from build123d import *

# Parameters (mm, degrees)
F5_R     = 30.5
F5_W     = 20
F5_H     = 15
F0_DEPTH = 80
F2_DEPTH = 1
F4_DEPTH = 1


with BuildPart() as f0:
    # F5 (on Top) → F0 (new body)
    with BuildSketch(Plane.XY):
        with BuildLine():
            ThreePointArc((-99, 0), (-66, 33), (-33, 0))
            Line((-33, 0), (-33, 50))
            Line((-33, 50), (-79, 50))
            Line((-79, 50), (-79, 35))
            Line((-79, 35), (-99, 35))
            Line((-99, 35), (-99, 0))
        make_face()
        with BuildLine():
            ThreePointArc((-99, 0), (-66, -33), (-33, 0))
            ThreePointArc((-33, 0), (-66, 33), (-99, 0))
        make_face()
        with Locations((-66, 0)):
            Circle(F5_R, mode=Mode.SUBTRACT)
        with Locations((-89, 42.5)):
            Rectangle(F5_W, F5_H)
    extrude(amount=F0_DEPTH)

    # F1 (on face) → F2 (join)
    with BuildSketch(Plane.YZ.offset(-33)):
        Polygon((33.663927, 32.829516), (33.663927, 57.098736), (2.563593, 75.054523), (2.563593, 51.653499), (2.563593, 14.865377), (18.11376, 5.887484), (19.11376, 6.464834), (33.663927, 14.865377), (33.663927, 15.595676), align=None)
        Polygon((4.563593, 51.165515), (4.563593, 71.590421), (31.663927, 55.944036), (31.663927, 53.944036), (31.663927, 46.022312), (31.663927, 43.27108), (31.663927, 32.829516), (31.663927, 16.020077), (18.11376, 8.196885), (4.563593, 16.020077), (4.563593, 32.829516), (4.563593, 35.912469), (4.563593, 36.259414), (4.563593, 38.259414), (4.563593, 49.165515), align=None, mode=Mode.SUBTRACT)
        Polygon((14.651485, 52.944283), (4.563593, 51.165515), (4.563593, 49.165515), (31.663927, 53.944036), (31.663927, 55.944036), (16.651485, 53.296937), align=None)
        Polygon((14.651485, 60.74453), (14.651485, 52.944283), (16.651485, 53.296937), (16.651485, 60.74453), (15.651485, 61.32188), align=None)
        Polygon((17.873782, 38.259414), (4.563593, 35.912469), (4.563593, 32.829516), (19.873782, 35.529115), (19.873782, 46.225284), (18.873782, 46.802635), (17.873782, 46.225284), align=None)
        Polygon((31.663927, 43.27108), (31.663927, 46.022312), (23.782982, 38.337872), (24.068827, 37.214549), (25.17923, 36.905919), align=None)
        Polygon((31.663927, 32.829516), (31.663927, 43.27108), (25.17923, 36.905919), (24.068827, 37.214549), align=None)
        Polygon((21.413582, 22.519643), (21.413582, 26.32995), (18.11376, 28.235103), (14.813938, 26.32995), (14.813938, 22.519643), (18.11376, 20.61449), align=None)
    extrude(amount=F2_DEPTH)

    # F3 (on face) → F4 (join)
    with BuildSketch(Plane(origin=(-99, 0, 0), x_dir=(0, -1, 0), z_dir=(-1, 0, 0))):
        Polygon((-33.316614, 46.639109), (-33.316614, 22.369889), (-2.216279, 4.414102), (-2.216279, 27.815126), (-2.216279, 64.603248), (-17.766446, 73.581141), (-18.766446, 73.003791), (-33.316614, 64.603248), (-33.316614, 63.872949), align=None)
        Polygon((-4.216279, 28.303109), (-4.216279, 7.878204), (-31.316614, 23.524589), (-31.316614, 25.524589), (-31.316614, 33.446313), (-31.316614, 36.197545), (-31.316614, 46.639109), (-31.316614, 63.448548), (-17.766446, 71.27174), (-4.216279, 63.448548), (-4.216279, 46.639109), (-4.216279, 43.556156), (-4.216279, 43.209211), (-4.216279, 41.209211), (-4.216279, 30.303109), align=None, mode=Mode.SUBTRACT)
        Polygon((-17.526468, 41.209211), (-4.216279, 43.556156), (-4.216279, 46.639109), (-19.526468, 43.939509), (-19.526468, 33.243341), (-18.526468, 32.66599), (-17.526468, 33.243341), align=None)
        Polygon((-31.316614, 36.197545), (-31.316614, 33.446313), (-23.435668, 41.130753), (-23.721513, 42.254076), (-24.831917, 42.562706), align=None)
        Polygon((-31.316614, 46.639109), (-31.316614, 36.197545), (-24.831917, 42.562706), (-23.721513, 42.254076), align=None)
        Polygon((-21.066269, 56.948982), (-21.066269, 53.138675), (-17.766446, 51.233521), (-14.466624, 53.138675), (-14.466624, 56.948982), (-17.766446, 58.854135), align=None)
        Polygon((-14.304171, 26.524342), (-4.216279, 28.303109), (-4.216279, 30.303109), (-31.316614, 25.524589), (-31.316614, 23.524589), (-16.304171, 26.171688), align=None)
        Polygon((-14.304171, 18.724095), (-14.304171, 26.524342), (-16.304171, 26.171688), (-16.304171, 18.724095), (-15.304171, 18.146745), align=None)
    extrude(amount=F4_DEPTH)


solid = f0.part
For this review, take the finished solid that the model builds, in its own axes (mm). A direction names the side the tool comes from. Coordinates: 2 decimals unless noted, no trailing zeros. Loops run counter-clockwise (first coordinate to the right, second up) from the corner with the lowest first, then second, coordinate; pieces in that order, holes last. Notation, with made-up numbers: (16.5, -9.5) - (38.5, -9.5) arc R21 ccw to (38.5, -1.5) - close; hole circle Ø2 at (-16.5, -21.5). An arc over 180 degrees is marked (long way). Return JSON: item names as keys, results as strings.
Item 1: For faces 1 (the flat face through (-32.51, 18.33, 65.95)), 2 (the flat face through (-99.49, 23.92, 24.83)), 3 (the flat face through (-32.51, 12.11, 34.16)), list the 3-axis set-ups (+Z, -Z, +X, -X, +Y, -Y) from which the entire face can be reached by the end or side of a thin tool; tool diameter is ignored.
Determined:
{"face 1": "+Z, +X, +Y", "face 2": "-X", "face 3": "+X"}
Item 2: Take a section at B-B (x = -75.5). Give the boundary of the cut face in (y, z).
Determined:
{"outline": "(-31.6, 0) - (-28.98, 0) - (-28.98, 80) - (-31.6, 80) - close; (28.98, 0) - (50, 0) - (50, 80) - (28.98, 80) - close"}
Item 3: Insertion check: pin 1 (0.5 mm diameter, centred on x = -99.5, z = 23, fed in from +Y); pin 2 (0.8 mm diameter, centred on x = -99.5, z = 29.5, fed in from -Y); pin 3 (0.5 mm diameter, centred on x = -32.5, z = 26.5, fed in from +Y). Each pin has a flat end and moves straight along its axis. Give the tip position at first contact, or say it passes through.
Determined:
{"pin 1": "stops at y = 33.32", "pin 2": "stops at y = 2.22", "pin 3": "stops at y = 33.66"}
Item 4: Mouldability with a two-part tool opening along Y and no side actions: class faces 4 (the flat face through (-32.5, 11.3, 37.1)), 5 (the flat face through (-99.49, 9.88, 69.03)), 6 (the flat face through (-99, 36, 39)) as pulls with the +Y half, pulls with the -Y half, needs draft (parallel to the pull), parting line crosses it, or undercut.
Determined:
{"face 4": "undercut", "face 5": "pulls with the -Y half", "face 6": "needs draft"}
Item 5: For line 1 (Y direction, x = -66, z = 34); line 2 (X direction, y = 42, z = 76); line 3 (Y direction, x = -43, z = 72), list the stretches that pass through material, from the lowest coordinate up.
Determined:
{"line 1": "y = -33 to -30.5, 30.5 to 50", "line 2": "x = -99 to -33", "line 3": "y = -23.66 to -20.03, 20.03 to 50"}
Item 6: Take a section at C-C (y = 44.5). Give the boundary of the cut face in (x, z), then the cut area to 3 significant figures.
Determined:
{"outline": "(-99, 0) - (-33, 0) - (-33, 80) - (-99, 80) - close", "area": "5,280 mm2"}
Item 7: Take a section at A-A (x = -66). Give the boundary of the cut face in (y, z), then the cut area to 3 significant figures.
Determined:
{"outline": "(-33, 0) - (-30.5, 0) - (-30.5, 80) - (-33, 80) - close; (30.5, 0) - (50, 0) - (50, 80) - (30.5, 80) - close", "area": "1,760 mm2"}
